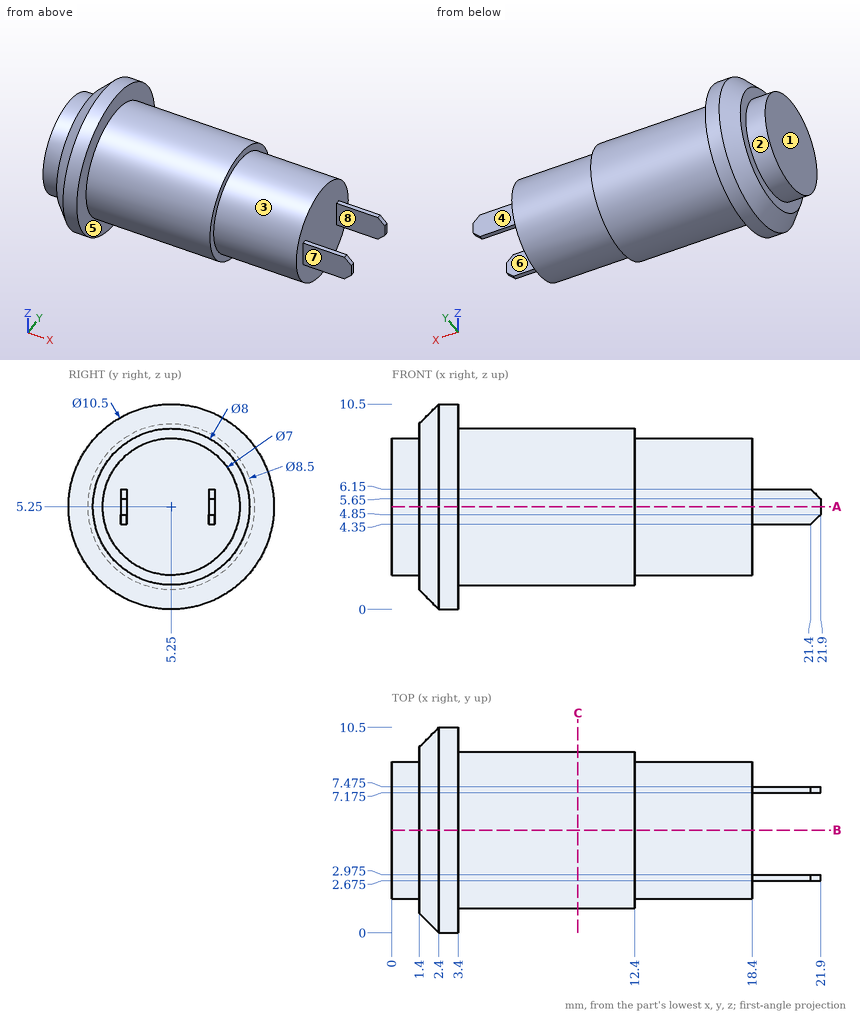
Geometry: see drawing. Coordinates: mm, zero at the bounding-box minimum. A direction names the side the tool comes from. Coordinates: 2 decimals unless noted, no trailing zeros. Order: outer loops, then holes, each group sorted by start corner. A loop starts at its lowest first (then second) coordinate and runs counter-clockwise, first axis right, second up. Notation, with made-up numbers: M 88,63.25 L 117,63.25 A22 cw 117,79.25 Z; hole C -40,58 d5. An arc over 180 degrees is marked long. Write each question's results on one line, items separated by ' | '. Start each with the question number.
1) Access query for the marked faces 1, 2, 3 and 4. Directions: +Z, -Z, +X, -X, +Y, -Y. A direction counts if a zero-diameter tool reaches every point of the face in a straight line with its end or side. Return the directions, or none.
2) Line query: line 1 (Y direction, x = 17.5, z = 5.25); line 2 (X direction, y = 3.5, z = 4.5); line 3 (X direction, y = 8.25, z = 3). Output: solid intervals per line, ascending. Write a range as from..to.
3) Section query B-B (y = 5.25). Return the cut outline in (x, z), plus the area to 3 significant figures.
4) Contact query for flat-ended pins moving along their axis: pin 1 Ø2 at (y, z) = (5, 6.5) entering from +X; pin 2 Ø6 at (x, z) = (19, 1.5) entering from -Y; pin 3 Ø4 at (x, z) = (19, 4.5) entering from +Y. Output: stop coordinate, or through.
5) Draft query along Y for the marked faces 5, 6, 7 and 8. Return one class per face: released by +Y, released by -Y, zero draft, split by the parting line, or undercut.
6) Section query C-C (x = 9.5). Return the cut outline in (y, z).
7) Section query A-A (z = 5.25). Return the cut outline in (x, y) (3 decimals).
Answers:
1) face 1: +Z, -Z, -X, +Y, -Y | face 2: -X | face 3: +X | face 4: +Z, -Z, +X, +Y
2) line 1: y = 1.75..8.75 | line 2: x = 0..18.4 | line 3: x = 1.4..12.4
3) outline: M 0,1.75 L 1.4,1.75 L 1.4,1 L 2.4,0 L 3.4,0 L 3.4,1.25 L 12.4,1.25 L 12.4,1.75 L 18.4,1.75 L 18.4,8.75 L 12.4,8.75 L 12.4,9.25 L 3.4,9.25 L 3.4,10.5 L 2.4,10.5 L 1.4,9.5 L 1.4,8.75 L 0,8.75 Z | area: 144 mm^2
4) pin 1: stops at x = 18.4 | pin 2: stops at y = 1.85 | pin 3: stops at y = 8.75
5) face 5: zero draft | face 6: undercut | face 7: released by -Y | face 8: undercut
6) outline: C 5.25,5.25 d8
7) outline: M 0,1.75 L 1.4,1.75 L 1.4,1 L 2.4,0 L 3.4,0 L 3.4,1.25 L 12.4,1.25 L 12.4,1.75 L 18.4,1.75 L 18.4,2.675 L 21.9,2.675 L 21.9,2.975 L 18.4,2.975 L 18.4,7.175 L 21.9,7.175 L 21.9,7.475 L 18.4,7.475 L 18.4,8.75 L 12.4,8.75 L 12.4,9.25 L 3.4,9.25 L 3.4,10.5 L 2.4,10.5 L 1.4,9.5 L 1.4,8.75 L 0,8.75 Z
